Autodesk Inventor part; units mm, degrees
ref_plane "YZ Plane" through (0, 0, 0) normal (1, 0, 0) x (0, 1, 0)
ref_plane "XZ Plane" through (0, 0, 0) normal (0, 1, 0) x (-1, 0, 0)
ref_plane "XY Plane" through (0, 0, 0) normal (0, 0, 1) x (1, 0, 0)
sketch "Sketch1" plane through (0, 0, 0) normal (0, 0, 1) x (1, 0, 0)
  arc A0 (0, 25) -> (0, -25) centre (0, 0) ccw
  arc A1 (500, -25) -> (500, 25) centre (500, 0) ccw
  line L0 (0, 25) -> (500, 25)
  line L1 (500, -25) -> (0, -25)
  arc A2 (0, 23) -> (0, -23) centre (0, 0) ccw
  arc A3 (500, -23) -> (500, 23) centre (500, 0) ccw
  line L2 (500, 0) -> (500, 23) construction
  line L3 (500, 0) -> (523, 0) construction
  line L4 (0, 23) -> (500, 23)
  line L5 (0, -23) -> (500, -23)
  dimension "D" = 50
  dimension "d2" = 50
  dimension "r" = 23
  dimension "d6" = 23
  dimension "d7" = 90
  dimension "L" = 500
extrude "Extrusion1" add sketch "Sketch1" against normal blind 200
sketch "Sketch2" plane through (0, 0, 0) normal (0, 0, 1) x (1, 0, 0)
  circle A0 centre (0, 0) radius 22.5
  arc A1 (500, -23) -> (500, 23) centre (500, 0) ccw construction
  circle A2 centre (500, 0) radius 22.5
  point P0 (300, -23)
  dimension "d" = 45
  dimension "d12" = 45
extrude "Extrusion2" add sketch "Sketch2" against normal blind 200
sketch "Sketch3" plane through (0, 0, 0) normal (0, 0, 1) x (1, 0, 0)
  arc A0 (5, 0) -> (-5, 0) centre (0, 0) ccw
  circle A1 centre (500, 0) radius 22.5 construction
  arc A2 (505, 0) -> (495, 0) centre (500, 0) ccw
  line L0 (5, 0) -> (5, -175)
  line L1 (5, -175) -> (-5, -175)
  line L2 (-5, -175) -> (-5, 0)
  line L3 (495, 0) -> (495, -175)
  line L4 (495, -175) -> (505, -175)
  line L5 (505, -175) -> (505, 0)
  dimension "altura" = 175
  dimension "d19" = 175
  dimension "d20" = 5
  dimension "d21" = 5
extrude "Extrusion3" add sketch "Sketch3" along normal blind 10
sketch "Sketch4" plane through (0, 0, -200) normal (0, 0, -1) x (-1, 0, 0)
  arc A0 (5, 0) -> (-5, 0) centre (0, 0) ccw
  arc A1 (5, 0) -> (-5, 0) centre (0, 0) ccw
  arc A2 (-495, 0) -> (-505, 0) centre (-500, 0) ccw
  arc A3 (-495, 0) -> (-505, 0) centre (-500, 0) ccw
  line L0 (-505, -175) -> (-505, 0)
  line L1 (-495, 0) -> (-495, -175)
  line L2 (-495, 0) -> (-495, -175)
  line L3 (-495, -175) -> (-505, -175)
  line L4 (-505, -175) -> (-505, 0)
  line L5 (5, -175) -> (-5, -175)
  line L6 (-5, 0) -> (-5, -175)
  line L7 (-5, -175) -> (5, -175)
  line L8 (5, -175) -> (5, 0)
  point P0 (-5, 0)
extrude "Extrusion4" add sketch "Sketch4" along normal blind 10
equation "\"d2\" = D"
equation "\"d6\" = r"
equation "\"d12\" = d"
equation "\"d19\" = altura"
properties part number "Banda"
Design review of the part built by this model. Coordinates are the model's own, in mm. A direction names the side the tool comes from. Give positions to 0.01 mm unless a question says otherwise; leave off trailing zeros. Order: outer loops, then holes, each group sorted by start corner. A loop starts at its lowest first (then second) coordinate and runs counter-clockwise, first axis right, second up.
1. Add section C-C, the plane x = 87. State the section outline as (y, z) points.
Solution:
outline: (-25, -200) - (-23, -200) - (-23, 0) - (-25, 0) - close; (23, -200) - (25, -200) - (25, 0) - (23, 0) - close
2. Mouldability with a two-part tool opening along Y and no side actions: class faces 4 (the flat face through (0, -84, 10)), 5 (the cylindrical face through (500, 5, -205)), 6 (the cylindrical face through (-22.994, 0.506, -98.6)) as +Y half, -Y half, draft (parallel to the pull), parting line (faces both ways), or undercut.
Solution:
face 4: draft
face 5: +Y half
face 6: undercut
3. To check wall thickness, follow L1, parallel to Y at x = 501.5, z = -40; L2, parallel to Y at x = 299, z = -156; L3, parallel to X at y = 15.5, z = -133.5. State the ranges of each line that lie inside material, in increasing order.
Solution:
L1: y = -24.95 to -22.95, -22.45 to 22.45, 22.95 to 24.95
L2: y = -25 to -23, 23 to 25
L3: x = -19.62 to -16.99, -16.31 to 16.31, 483.69 to 516.31, 516.99 to 519.62
4. For pin 1 Ø13.5 at (x, y) = (499, 8) entering from -Z; pin 2 Ø8 at (y, z) = (-70.5, 3) entering from -X; pin 3 Ø6 at (y, z) = (-17.5, -77.5) entering from -X; pin 4 Ø1 at (x, z) = (315.5, -37) entering from -Y, all flat-tipped, find the tip position at first contact; note any pin that passes through.
Solution:
pin 1: stops at z = -210
pin 2: stops at x = -5
pin 3: stops at x = -20.37
pin 4: stops at y = -25
5. Tool access review of faces 1 (the cylindrical face through (0, 5, 5)), 2 (the flat face through (0, -175, 5)), 3 (the flat face through (500, -99, 0)): name each direction out of +Z, -Z, +X, -X, +Y, -Y from which nothing blocks a thin tool from reaching the whole face with its end or side.
Solution:
face 1: +Z, +Y
face 2: +Z, -Z, +X, -X, -Y
face 3: +X, -X, -Y
6. Add section B-B, the plane y = -84. State the section outline as (x, z) points, then the cut area to 3 significant figures.
Solution:
outline: (-5, -210) - (5, -210) - (5, -200) - (-5, -200) - close; (-5, 0) - (5, 0) - (5, 10) - (-5, 10) - close; (495, -210) - (505, -210) - (505, -200) - (495, -200) - close; (495, 0) - (505, 0) - (505, 10) - (495, 10) - close
area: 400 mm2
7. Add section A-A, the plane z = -66. State the section outline as (x, y) points, then the cut area to 3 significant figures.
Solution:
outline: circle Ø45 at (0, 0); (0, -25) - (500, -25) arc R25 ccw to (500, 25) - (0, 25) arc R25 ccw to start; circle Ø45 at (500, 0); hole (0, -23) - (500, -23) arc R23 ccw to (500, 23) - (0, 23) arc R23 ccw to start
area: 5,480 mm2
